Geometry: final body of the model. Coordinates: model frame, mm. A direction names the side the tool comes from. Give positions to 0.01 mm unless a question says otherwise; leave off trailing zeros. Loops run counter-clockwise (first coordinate to the right, second up) from the corner with the lowest first, then second, coordinate; pieces in that order, holes last. Notation, with made-up numbers: (5.5, 80.5) -> (54.5, 80.5) arc R22 ccw to (54.5, 105.5) -> close; hole circle Ø1 at (70.5, 21). An arc over 180 degrees is marked (long way). Answer in a Markdown table with one row per item. Add a question column.
1) Section query B-B (x = -16). Return the cut outline in (y, z) (1 decimal).
2) First-contact query: P1, Ø5, axis at x = -23.5, z = 19, coming from the -Y side. Flat tip, straight axial feed; report the tip coordinate or a pass-through.
3) Line query: line 1 (Z direction, x = -37.5, y = 9.5); line 2 (X direction, y = 15, z = 27); line 3 (Y direction, x = 36, z = -14) (3 decimals). Output: solid intervals per line, ascending. Write a range as from..to.
4) Draft query along Z for faces 3 (the flat face through (-1, 41.275, 0)), 4 (the cylindrical face through (-4.725, 39.71, -3.583)), 5 (the cylindrical face through (-43.535, 19.639, 30.097)). Return one class per face: +Z half, -Z half, draft (parallel to the pull), parting line (faces both ways), or undercut.
5) Section query A-A (y = 27.5). Return the cut outline in (x, z).
6) Access query for faces 1 (the cylindrical face through (0.597, 37.336, 28.549)), 2 (the cylindrical face through (7.975, 39.71, -3.583)). Directions: +Z, -Z, +X, -X, +Y, -Y. A direction counts if a zero-diameter tool reaches every point of the face in a straight line with its end or side. Return the directions, or none.
7) Section query C-C (z = -7). Return the cut outline in (x, y) (1 decimal).
```python
from build123d import *

# Parameters (mm, degrees)
SKETCH3_W           = 88.519
SKETCH3_H           = 61.722
BOSS_EXTRUDE2_DEPTH = 41.275
SKETCH1_W           = 85.344
SKETCH1_H           = 58.547
CUT_EXTRUDE1_DEPTH  = 38.1
FILLET2_R           = 2.54
SKETCH6_R           = 1.5875
CUT_EXTRUDE4_DEPTH  = 42.275
FILLET3_R           = 2.54


with BuildPart() as part:
    # Sketch3 → Boss-Extrude2 (new body)
    with BuildSketch(Plane(origin=(0, 0, 0), x_dir=(1, 0, 0), z_dir=(0, 1, 0))):
        Rectangle(SKETCH3_W, SKETCH3_H)
    extrude(amount=BOSS_EXTRUDE2_DEPTH)

    # Sketch1 → Cut-Extrude1 (cut)
    with BuildSketch(Plane(origin=(0, 0, 0), x_dir=(1, 0, 0), z_dir=(0, 1, 0))):
        Rectangle(SKETCH1_W, SKETCH1_H)
    extrude(amount=CUT_EXTRUDE1_DEPTH, mode=Mode.SUBTRACT)

    # Fillet2
    fillet2_edges = [part.edges().sort_by_distance(p)[0] for p in [
        (-44.2595, 41.275, 0),
        (0, 41.275, 30.861),
        (44.2595, 41.275, 0),
        (0, 41.275, -30.861),
        (44.2595, 20.6375, 30.861),
        (-44.2595, 20.6375, 30.861),
        (-44.2595, 20.6375, -30.861),
        (44.2595, 20.6375, -30.861),
    ]]
    fillet(fillet2_edges, radius=FILLET2_R)

    # Sketch6 → Cut-Extrude4 (cut, through all)
    with BuildSketch(Plane(origin=(0, 41.275, 0), x_dir=(1, 0, 0), z_dir=(0, 1, 0))):
        with Locations(Location((-9.525, -3.1115, 0), (0, 0, 270))):  # turned: the seam where the file's is
            Circle(SKETCH6_R)
        with Locations(Location((-3.175, -3.1115, 0), (0, 0, 270))):  # turned: the seam where the file's is
            Circle(SKETCH6_R)
        with Locations(Location((3.175, -3.1115, 0), (0, 0, 270))):  # turned: the seam where the file's is
            Circle(SKETCH6_R)
        with Locations(Location((9.525, -3.1115, 0), (0, 0, 270))):  # turned: the seam where the file's is
            Circle(SKETCH6_R)
        with Locations(Location((-9.525, 3.2385, 0), (0, 0, 270))):  # turned: the seam where the file's is
            Circle(SKETCH6_R)
        with Locations(Location((-3.175, 3.2385, 0), (0, 0, 270))):  # turned: the seam where the file's is
            Circle(SKETCH6_R)
        with Locations(Location((3.175, 3.2385, 0), (0, 0, 270))):  # turned: the seam where the file's is
            Circle(SKETCH6_R)
        with Locations(Location((9.525, 3.2385, 0), (0, 0, 270))):  # turned: the seam where the file's is
            Circle(SKETCH6_R)
    extrude(amount=-CUT_EXTRUDE4_DEPTH, mode=Mode.SUBTRACT)

    # Fillet3
    fillet3_edges = [part.edges().sort_by_distance(p)[0] for p in [
        (42.672, 38.1, 0),
        (0, 38.1, -29.2735),
        (-42.672, 38.1, 0),
        (0, 38.1, 29.2735),
    ]]
    fillet(fillet3_edges, radius=FILLET3_R)


solid = part.part
```
Evaluation:
| question | item | result |
|---|---|---|
| 1 | outline | (0, -30.9) -> (38.7, -30.9) arc R2.5 ccw to (41.3, -28.3) -> (41.3, 28.3) arc R2.5 ccw to (38.7, 30.9) -> (0, 30.9) -> (0, 29.3) -> (35.6, 29.3) arc R2.5 cw to (38.1, 26.7) -> (38.1, -26.7) arc R2.5 cw to (35.6, -29.3) -> (0, -29.3) -> close |
| 2 | P1 | y = 38.1 |
| 3 | line 1 | -30.86..-29.27, 29.27..30.86 |
| 3 | line 2 | -44.26..-42.67, 42.67..44.26 |
| 3 | line 3 | 38.1..41.275 |
| 4 | face 3 | draft |
| 4 | face 4 | undercut |
| 4 | face 5 | +Z half |
| 5 | outline | (-44.26, -28.32) arc R2.54 ccw to (-41.72, -30.86) -> (41.72, -30.86) arc R2.54 ccw to (44.26, -28.32) -> (44.26, 28.32) arc R2.54 ccw to (41.72, 30.86) -> (-41.72, 30.86) arc R2.54 ccw to (-44.26, 28.32) -> close; hole (-42.67, -29.27) -> (42.67, -29.27) -> (42.67, 29.27) -> (-42.67, 29.27) -> close |
| 6 | face 1 | -Y |
| 6 | face 2 | +Y, -Y |
| 7 | outline | (-44.3, 0) -> (-42.7, 0) -> (-42.7, 35.6) arc R2.5 cw to (-40.1, 38.1) -> (40.1, 38.1) arc R2.5 cw to (42.7, 35.6) -> (42.7, 0) -> (44.3, 0) -> (44.3, 38.7) arc R2.5 ccw to (41.7, 41.3) -> (-41.7, 41.3) arc R2.5 ccw to (-44.3, 38.7) -> close |
